Check sheet for the drawn part. Datum: minimum x, y, z corner. Units: mm. Give positions to 0.01 mm unless a question says otherwise; leave off trailing zeros. Order: outer loops, then holes, each group sorted by start corner. A loop starts at its lowest first (then second) coordinate and runs counter-clockwise, first axis right, second up. Notation, with made-up numbers: (47, -36.5) -> (59, -36.5) arc R15 cw to (59, -12.5) -> close; hole circle Ø10 at (87.5, 48.5). An arc over 180 degrees is marked (long way). Answer in a Markdown table with one row per item. Add a question column.
(1) Cross-section at C-C (z = 34.5). Record the cut outline in (x, y) (1 decimal).
(2) Cross-section at D-D (z = 8.5). Record the cut outline in (x, y) (1 decimal).
(3) Go/stop test with flat-tipped pins: pin 1 (0.9 mm diameter, centred on y = 1.5, z = 33, fed in from -X) (1 decimal); pin 2 (1.5 mm diameter, centred on x = 37, y = 1.5, fed in from -Z); pin 3 (0.9 mm diameter, centred on x = 1, y = 1, fed in from +Z). Record where each tip stops, or that it passes through.
(4) Thickness scan on L1, parallel to Z at x = 16, y = 0.35 (1 decimal); L2, parallel to X at y = 1.9, z = 34 (1 decimal); L3, parallel to X at y = 1.85, z = 18 (1 decimal). Record the ranges inside material, lowest first. Write a range as [from, to].
(5) Cross-section at A-A (x = 23.5). Record the cut outline in (y, z) (1 decimal).
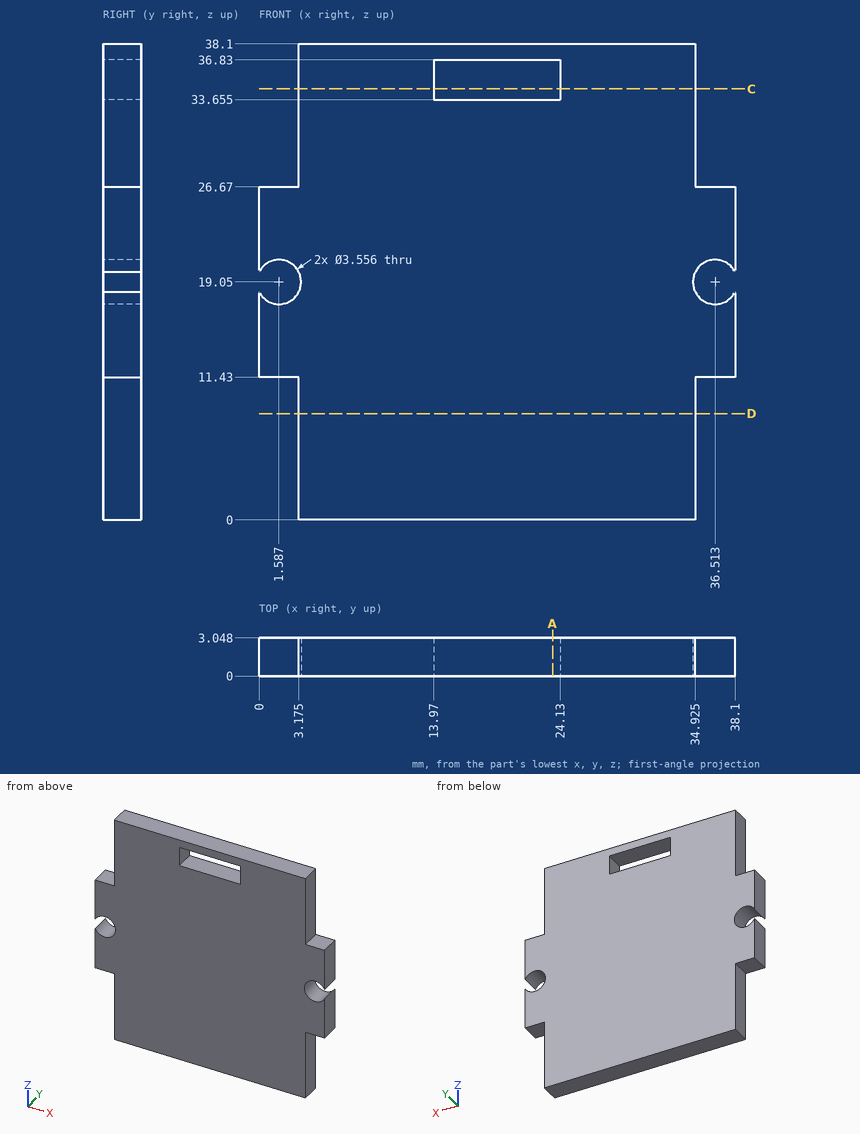
Answer below:
| question | item | result |
|---|---|---|
| 1 | outline | (3.2, 0) -> (14, 0) -> (14, 3) -> (3.2, 3) -> close; (24.1, 0) -> (34.9, 0) -> (34.9, 3) -> (24.1, 3) -> close |
| 2 | outline | (3.2, 0) -> (34.9, 0) -> (34.9, 3) -> (3.2, 3) -> close |
| 3 | pin 1 | stops at x = 3.2 |
| 3 | pin 2 | stops at z = 11.43 |
| 3 | pin 3 | stops at z = 26.67 |
| 4 | L1 | z = [0, 33.7], [36.8, 38.1] |
| 4 | L2 | x = [3.2, 14], [24.1, 34.9] |
| 4 | L3 | x = [0, 0.2], [3, 35.1], [37.9, 38.1] |
| 5 | outline | (0, 0) -> (3, 0) -> (3, 33.7) -> (0, 33.7) -> close; (0, 36.8) -> (3, 36.8) -> (3, 38.1) -> (0, 38.1) -> close |
